```python
from build123d import *

# Parameters (mm, degrees)
F0_W     = 36
F0_H     = 36
F1_DEPTH = 56
F2_W     = 21
F2_H     = 41
F3_DEPTH = 28
F4_W     = 21
F4_H     = 20.5
F5_DEPTH = 70
F6_R     = 2.6
F7_DEPTH = 20
F8_R     = 4.35
F9_DEPTH = 5.5


with BuildPart() as f1:
    # F0 (on Top) → F1 (new body)
    with BuildSketch(Plane.XY):
        with Locations((18, 18)):
            Rectangle(F0_W, F0_H)
    extrude(amount=F1_DEPTH)

    # F2 (on face) → F3 (cut)
    with BuildSketch(Plane(origin=(0, 0, 0), x_dir=(0, -1, 0), z_dir=(-1, 0, 0))):
        with Locations((-18, 28)):
            Rectangle(F2_W, F2_H)
    extrude(amount=-F3_DEPTH, mode=Mode.SUBTRACT)

    # F4 (on face) → F5 (cut)
    with BuildSketch(Plane(origin=(0, 0, 0), x_dir=(0, -1, 0), z_dir=(-1, 0, 0))):
        with Locations((-18, 38.25)):
            Rectangle(F4_W, F4_H)
    extrude(amount=-F5_DEPTH, mode=Mode.SUBTRACT)

    # F6 (on face) → F7 (cut)
    with BuildSketch(Plane.XZ):
        with Locations((18, 38)):
            Circle(F6_R)
        with Locations((14, 18)):
            Circle(F6_R)
    extrude(amount=-F7_DEPTH, mode=Mode.SUBTRACT)

    # F8 (on face) → F9 (cut)
    with BuildSketch(Plane.XZ):
        with Locations((18, 38)):
            Circle(F8_R)
        with Locations((14, 18)):
            Circle(F8_R)
    extrude(amount=-F9_DEPTH, mode=Mode.SUBTRACT)


solid = f1.part
```
Can you work these out from the model? Positions are in its coordinate system, mm. A direction names the side the tool comes from. Coordinates: 2 decimals unless noted, no trailing zeros. Loops run counter-clockwise (first coordinate to the right, second up) from the corner with the lowest first, then second, coordinate; pieces in that order, holes last. Notation, with made-up numbers: M -21.5,28.5 L -17.5,28.5 A10 cw -17.5,44.5 Z; hole C 50,23 d9. An arc over 180 degrees is marked long. Put each result on its own line as item: value. Start each with the question number.
(1) Which directions (+Z, -Z, +X, -X, +Y, -Y) give clear straight access to the entire face, cutting with the end or side of a thin tool? Please do faces 1 (the face through (14, 18, 7.5)), 2 (the face through (18, 18, 48.5)), 3 (the face through (19.2, 6.486, 35.693)).
(2) Imagine slicing it at B-B on z = 18. List the corners of the cut face in (x, y) for me.
(3) Imagine slicing it at C-C on x = 33. List the corners of the cut face in (y, z) for me, and give its area (3 significant figures).
(4) We'd pull the mould along Y, two halves only. Please class faces 4 (the face through (16, 5.5, 16)), 5 (the face through (18, 7.5, 28)), 6 (the face through (22.15, 2.71, 39.31)): +Y half, -Y half, draft (parallel to the pull), parting line (faces both ways), or undercut.
(5) Imagine slicing it at A-A on z = 38. List the corners of the cut face in (x, y) for me.
(6) I need wall thicknesses on probe 1 along Z at (x, y) = (25.5, 16); probe 2 along Y at (x, z) = (25, 19.5); probe 3 along Z at (x, y) = (32, 9.5). Which ranges of each line are inside material? Lowest first, please.
(7) Imagine slicing it at D-D on y = 18.5. List the corners of the cut face in (x, z) for me.
(8) Will these pins go through, and if not, where does the flat tip stop? pin 1 Ø3 at (x, z) = (14, 18) entering from -Y; pin 2 Ø7 at (x, z) = (18, 38) entering from -Y; pin 3 Ø6 at (y, z) = (20, 19) entering from -X.
Worked answers:
1. face 1: -X
1. face 2: +X, -X
1. face 3: -Y
2. outline: M 0,0 L 9.65,0 L 9.65,5.5 L 11.4,5.5 L 11.4,7.5 L 0,7.5 Z; M 0,28.5 L 28,28.5 L 28,7.5 L 16.6,7.5 L 16.6,5.5 L 18.35,5.5 L 18.35,0 L 36,0 L 36,36 L 0,36 Z
3. outline: M 0,0 L 36,0 L 36,56 L 0,56 Z; hole M 7.5,28 L 28.5,28 L 28.5,48.5 L 7.5,48.5 Z
3. area: 1,590 mm2
4. face 4: -Y half
4. face 5: undercut
4. face 6: draft
5. outline: M 0,0 L 13.65,0 L 13.65,5.5 L 15.4,5.5 L 15.4,7.5 L 0,7.5 Z; M 0,28.5 L 36,28.5 L 36,36 L 0,36 Z; M 20.6,5.5 L 22.35,5.5 L 22.35,0 L 36,0 L 36,7.5 L 20.6,7.5 Z
6. probe 1: z = 0 to 7.5, 48.5 to 56
6. probe 2: y = 0 to 7.5, 28.5 to 36
6. probe 3: z = 0 to 28, 48.5 to 56
7. outline: M 0,0 L 36,0 L 36,28 L 28,28 L 28,7.5 L 0,7.5 Z; M 0,48.5 L 36,48.5 L 36,56 L 0,56 Z
8. pin 1: stops at y = 28.5
8. pin 2: stops at y = 5.5
8. pin 3: stops at x = 28
